Autodesk Inventor part; units mm, degrees
ref_plane "YZ Plane" through (0, 0, 0) normal (1, 0, 0) x (0, 1, 0)
ref_plane "XZ Plane" through (0, 0, 0) normal (0, 1, 0) x (-1, 0, 0)
ref_plane "XY Plane" through (0, 0, 0) normal (0, 0, 1) x (1, 0, 0)
sketch "Sketch1" plane through (0, 0, 0) normal (0, 1, 0) x (-1, 0, 0)
  circle A0 centre (-55, 111.5) radius 1.6
  circle A1 centre (-55.4645, -12) radius 1.6
  circle A2 centre (8, -12) radius 1.6
  circle A3 centre (8, 111.5) radius 1.6
  arc A4 (-67, 109) -> (-69, 107) centre (-67, 107) ccw
  line L0 (-69, 107) -> (-69, -7.5)
  arc A5 (-69, -7.5) -> (-67, -9.5) centre (-67, -7.5) ccw
  line L1 (-67, -9.5) -> (-64, -9.5)
  line L2 (-59, -14.5) -> (-64, -9.5)
  line L3 (-51, -14.5) -> (-59, -14.5)
  line L4 (-46, -9.5) -> (-51, -14.5)
  line L5 (-46, -9.5) -> (-1, -9.5)
  line L6 (-1, -9.5) -> (4, -14.5)
  line L7 (4, -14.5) -> (12, -14.5)
  line L8 (12, -14.5) -> (17, -9.5)
  line L9 (17, -9.5) -> (20, -9.5)
  arc A6 (20, -9.5) -> (22, -7.5) centre (20, -7.5) ccw
  line L10 (22, -7.5) -> (22, 107)
  arc A7 (22, 107) -> (20, 109) centre (20, 107) ccw
  line L11 (20, 109) -> (17, 109)
  line L12 (17, 109) -> (12, 114)
  line L13 (12, 114) -> (4, 114)
  line L14 (4, 114) -> (-1, 109)
  line L15 (-1, 109) -> (-46, 109)
  line L16 (-46, 109) -> (-51, 114)
  line L17 (-51, 114) -> (-59, 114)
  line L18 (-59, 114) -> (-64, 109)
  line L19 (-64, 109) -> (-67, 109)
  point P0 (0, 0)
  point P1 (0, 0)
extrude "Extrusion1" add sketch "Sketch1" along normal blind 10
sketch "Sketch4" plane through (0, 0, 0) normal (0, -1, 0) x (1, 0, 0)
  line L0 (65, 105) -> (-18, 105)
  line L1 (-18, 105) -> (-18, -5.5)
  line L2 (-18, -5.5) -> (65, -5.5)
  line L3 (65, -5.5) -> (65, 105)
  line L4 (1, 109) -> (46, 109)
  line L5 (46, -9.5) -> (1, -9.5)
  line L6 (-22, -7.5) -> (-22, 107)
  line L7 (69, 107) -> (69, -7.5)
  point P0 (0, 0)
  dimension "d2" = 4
  dimension "d3" = 4
  dimension "d4" = 4
  dimension "d5" = 4
extrude "Extrusion2" cut sketch "Sketch4" against normal blind 6
fillet "Fillet1" radius 2 4 edges at (65, 3, 105) (-18, 3, 105) (65, 3, -5.5) (-18, 3, -5.5)
sketch "Sketch5" plane through (0, 10, 0) normal (0, 1, 0) x (1, 0, 0)
  line L0 (64, -109) -> (67, -109)
  line L1 (-40.3504, -169.2964) -> (66.299, -169.2964)
  line L2 (66.299, -169.2964) -> (66.299, -109)
  line L3 (66.299, -109) -> (-40.3504, -109)
  line L4 (-40.3504, -109) -> (-40.3504, -169.2964)
  line L5 (-53.7547, 54.3444) -> (65.5201, 54.3444)
  line L6 (65.5201, 54.3444) -> (65.5201, 9.5)
  line L7 (65.5201, 9.5) -> (-53.7547, 9.5)
  line L8 (-53.7547, 9.5) -> (-53.7547, 54.3444)
  point P0 (0, 0)
extrude "Extrusion3" cut sketch "Sketch5" against normal blind 6
sketch "Sketch6" plane through (0, 0, 0) normal (0, -1, 0) x (1, 0, 0)
  line L0 (67.5, 107.5) -> (-20.5, 107.5)
  line L1 (-20.5, 107.5) -> (-20.5, -8)
  line L2 (-20.5, -8) -> (67.5, -8)
  line L3 (67.5, -8) -> (67.5, 107.5)
  line L4 (67, -9.5) -> (-20, -9.5)
  line L5 (-22, -7.5) -> (-22, 107)
  line L6 (69, 107) -> (69, -7.5)
  line L7 (-20, 109) -> (67, 109)
  line L8 (66.5, 106.5) -> (-19.5, 106.5)
  line L9 (-19.5, 106.5) -> (-19.5, -7)
  line L10 (-19.5, -7) -> (66.5, -7)
  line L11 (66.5, -7) -> (66.5, 106.5)
  point P0 (0, 0)
  dimension "d11" = 1.5
  dimension "d12" = 1.5
  dimension "d13" = 1.5
  dimension "d14" = 1.5
  dimension "d15" = 1
  dimension "d16" = 1
  dimension "d17" = 1
  dimension "d18" = 1
extrude "Extrusion4" add sketch "Sketch6" along normal blind 3
fillet "Fillet2" radius 2 8 edges at (-20.5, -1.5, 107.5) (67.5, -1.5, 107.5) (66.5, -1.5, 106.5) (-19.5, -1.5, 106.5) (-20.5, -1.5, -8) (-19.5, -1.5, -7) (67.5, -1.5, -8) (66.5, -1.5, -7)
properties part number "Top"
Source: CAD feature listing. Evaluate the final solid. Frame: model axes, mm. A direction names the side the tool comes from. Coordinates: 2 decimals unless noted, no trailing zeros. Write each loop counter-clockwise with the first axis right and the second up, starting at its lowest first coordinate (ties: lowest second). Pieces come first, ordered by that corner, then holes. Notation, with made-up numbers: (34, -4.5) -> (72, -4.5) arc R16 ccw to (72, 13.5) -> close; hole circle Ø6 at (59.25, -9.75). An arc over 180 degrees is marked (long way). Return JSON: item names as keys, results as strings. Group by question number.
1) Ray query, line 1 along Z through (x, y) = (-8, 3.15); line 2 along X through (y, z) = (1.75, 8); line 3 along X through (y, z) = (-2, 25.5). Return the intervals inside material, ascending.
2) Mould query, pull axis Z, two halves, no side actions, for faces 1 (the face through (-6.82, 1.97, -13.08)), 2 (the face through (55, 4, -10)), 3 (the face through (48, 2, 111)). Classes: +Z half, -Z half, draft (parallel to the pull), parting line (faces both ways), or undercut.
3) Section query B-B, the plane x = -8. Return loops of the section in (y, z), plus the area to 3 significant figures.
4) Set-up query: faces 4 (the face through (24, -1, 107.5)), 5 (the face through (54.9, 4, 109.2)), 6 (the face through (-19.5, -1, 51)). Return all of +Z, -Z, +X, -X, +Y, -Y with unobstructed straight access to the full face (end or side cutting, diameter ignored); none if empty.
5) Contact query for flat-ended pins moving along their axis: P1, Ø0.9, axis at x = 36, y = -2, coming from the -Z side; P2, Ø1, axis at x = 0, y = 7, coming from the -Z side; P3, Ø4, axis at x = -1.5, y = 0.5, coming from the +Z side; P4, Ø2.5, axis at x = 55, z = 111.5, coming from the -Y side. Output: stop coordinate, or through.
6) Section query D-D, the plane x = 4. Return loops of the section in (y, z), plus the area to 3 significant figures.
7) Section query A-A, the plane z = -12. Return loops of the section in (x, y), plus the area to 3 significant figures.
8) Section query C-C, the plane z = 82.5. Return loops of the section in (x, y), plus the area to 3 significant figures.
From the geometry:
{
 "1": {"line 1": "-14.5 to -13.6, -10.4 to -5.5, 105 to 109.9, 113.1 to 114", "line 2": "-22 to -18, 65 to 69", "line 3": "-20.5 to -19.5, 66.5 to 67.5"},
 "2": {"face 1": "undercut", "face 2": "draft", "face 3": "+Z half"},
 "3": {"outline": "(-3, -8) -> (0, -8) -> (0, -10.4) -> (4, -10.4) -> (4, -9.5) -> (10, -9.5) -> (10, 109) -> (4, 109) -> (4, 109.9) -> (0, 109.9) -> (0, 107.5) -> (-3, 107.5) -> (-3, 106.5) -> (0, 106.5) -> (0, 105) -> (6, 105) -> (6, -5.5) -> (0, -5.5) -> (0, -7) -> (-3, -7) -> close; (0, -14.5) -> (4, -14.5) -> (4, -13.6) -> (0, -13.6) -> close; (0, 113.1) -> (4, 113.1) -> (4, 114) -> (0, 114) -> close", "area": "542 mm²"},
 "4": {"face 4": "+Z, +X, -X, -Y", "face 5": "+Z, +X, -X, +Y", "face 6": "-Y"},
 "5": {"P1": "z = -8", "P2": "z = -9.5", "P3": "z = 113.5", "P4": "through"},
 "6": {"outline": "(-3, -8) -> (0, -8) -> (0, -9.5) -> (10, -9.5) -> (10, 109) -> (0, 109) -> (0, 107.5) -> (-3, 107.5) -> (-3, 106.5) -> (0, 106.5) -> (0, 105) -> (6, 105) -> (6, -5.5) -> (0, -5.5) -> (0, -7) -> (-3, -7) -> close", "area": "528 mm²"},
 "7": {"outline": "(-14.5, 0) -> (-9.6, 0) -> (-9.6, 4) -> (-14.5, 4) -> close; (-6.4, 0) -> (-1.5, 0) -> (-1.5, 4) -> (-6.4, 4) -> close; (48.5, 0) -> (53.86, 0) -> (53.86, 4) -> (48.5, 4) -> close; (57.06, 0) -> (61.5, 0) -> (61.5, 4) -> (57.06, 4) -> close", "area": "78.4 mm²"},
 "8": {"outline": "(-22, 0) -> (-20.5, 0) -> (-20.5, -3) -> (-19.5, -3) -> (-19.5, 0) -> (-18, 0) -> (-18, 6) -> (65, 6) -> (65, 0) -> (66.5, 0) -> (66.5, -3) -> (67.5, -3) -> (67.5, 0) -> (69, 0) -> (69, 10) -> (-22, 10) -> close", "area": "418 mm²"}
}
